The model under review builds one solid part; all positions refer to its coordinate system, in mm. Face numbers are marked on the shaded views. A direction names the side the tool comes from. Round coordinates to 2 decimals unless told otherwise and drop trailing zeros. Write each loop counter-clockwise with the first axis right and the second up, starting at its lowest first coordinate (ties: lowest second). Pieces come first, ordered by that corner, then holes. Notation, with made-up numbers: (76.25, 57) -> (97.25, 57) arc R25 cw to (97.25, 74) -> close; hole circle Ø10 at (-20, 84.25). An arc over 180 degrees is marked (long way). Answer in a Markdown table with one row per item. Add a question column.
```python
from build123d import *

# Parameters (mm, degrees)
SKETCH1_W           = 11.5
SKETCH1_H           = 9
SKETCH1_R           = 1.6
SKETCH1_H_2         = 3
BOSS_EXTRUDE1_DEPTH = 3
SKETCH1_4_W         = 11.5
SKETCH1_4_H         = 3
BOSS_EXTRUDE2_DEPTH = 12
SKETCH1_5_R         = 1.6
CUT_EXTRUDE1_DEPTH  = 2.2
SKETCH1_6_R         = 1.6
CUT_EXTRUDE2_DEPTH  = 21.5
CUT_EXTRUDE3_DEPTH  = 2.2
CUT_EXTRUDE4_DEPTH  = 19.901058171


with BuildPart() as part:
    # Sketch1 → Boss-Extrude1 (new body)
    # profile 1 of 4: a face of its own
    with BuildSketch(Plane(origin=(0, 0, 0), x_dir=(1, 0, 0), z_dir=(0, 1, 0))):
        with Locations((5.75, 7.5)):
            Rectangle(SKETCH1_W, SKETCH1_H)
        Polygon((10.695041723, 7), (8.847520861, 3.8), (5.152479139, 3.8), (3.304958277, 7), (5.152479139, 10.2), (8.847520861, 10.2), align=None, mode=Mode.SUBTRACT)
    # profile 2 of 4: a face of its own
    with BuildSketch(Plane(origin=(0, 0, 0), x_dir=(1, 0, 0), z_dir=(0, 1, 0))):
        Polygon((3.304958277, 7), (5.152479139, 3.8), (8.847520861, 3.8), (10.695041723, 7), (8.847520861, 10.2), (5.152479139, 10.2), align=None)
        with Locations((7, 7)):
            Circle(SKETCH1_R, mode=Mode.SUBTRACT)
    # profile 3 of 4: a face of its own
    with BuildSketch(Plane(origin=(0, 0, 0), x_dir=(1, 0, 0), z_dir=(0, 1, 0))):
        with Locations((7, 7)):
            Circle(SKETCH1_R)
    # profile 4 of 4: a face of its own
    with BuildSketch(Plane(origin=(0, 0, 0), x_dir=(1, 0, 0), z_dir=(0, 1, 0))):
        with Locations((5.75, 1.5)):
            Rectangle(SKETCH1_W, SKETCH1_H_2)
    extrude(amount=BOSS_EXTRUDE1_DEPTH)

    # Sketch1_4 → Boss-Extrude2 (add)
    with BuildSketch(Plane(origin=(0, 0, 0), x_dir=(1, 0, 0), z_dir=(0, 1, 0))):
        with Locations((5.75, 1.5)):
            Rectangle(SKETCH1_4_W, SKETCH1_4_H)
    extrude(amount=-BOSS_EXTRUDE2_DEPTH)

    # Sketch1_5 → Cut-Extrude1 (cut)
    with BuildSketch(Plane(origin=(0, 0, 0), x_dir=(1, 0, 0), z_dir=(0, 1, 0))):
        Polygon((3.304958277, 7), (5.152479139, 3.8), (8.847520861, 3.8), (10.695041723, 7), (8.847520861, 10.2), (5.152479139, 10.2), align=None)
        with Locations(Location((7, 7, 0), (0, 0, 270))):
            Circle(SKETCH1_5_R, mode=Mode.SUBTRACT)
    extrude(amount=CUT_EXTRUDE1_DEPTH, mode=Mode.SUBTRACT)

    # Sketch1_6 → Cut-Extrude2 (cut, through all)
    with BuildSketch(Plane(origin=(0, 0, 0), x_dir=(1, 0, 0), z_dir=(0, 1, 0))):
        with Locations(Location((7, 7, 0), (0, 0, 270))):
            Circle(SKETCH1_6_R)
    extrude(amount=CUT_EXTRUDE2_DEPTH, mode=Mode.SUBTRACT)

    # Sketch3 → Cut-Extrude3 (cut)
    with BuildSketch(Plane(origin=(0, 0, -3), x_dir=(-1, 0, 0), z_dir=(0, 0, -1))):
        with BuildLine():
            Line((-0.304958277, -7), (-2.3, -7))
            ThreePointArc((-2.3, -7), (-4, -8.7), (-5.7, -7))
            Line((-5.7, -7), (-7.695041723, -7))
            Line((-7.695041723, -7), (-5.847520861, -10.2))
            Line((-5.847520861, -10.2), (-2.152479139, -10.2))
            Line((-2.152479139, -10.2), (-0.304958277, -7))
        make_face()
        with BuildLine():
            ThreePointArc((-5.7, -7), (-4, -5.3), (-2.3, -7))
            Line((-2.3, -7), (-0.304958277, -7))
            Line((-0.304958277, -7), (-2.152479139, -3.8))
            Line((-2.152479139, -3.8), (-5.847520861, -3.8))
            Line((-5.847520861, -3.8), (-7.695041723, -7))
            Line((-7.695041723, -7), (-5.7, -7))
        make_face()
    extrude(amount=-CUT_EXTRUDE3_DEPTH, mode=Mode.SUBTRACT)

    # Sketch3_3 → Cut-Extrude4 (cut, through all)
    with BuildSketch(Plane(origin=(0, 0, -3), x_dir=(-1, 0, 0), z_dir=(0, 0, -1))):
        with BuildLine():
            ThreePointArc((-5.7, -7), (-4, -8.7), (-2.3, -7))
            Line((-2.3, -7), (-5.7, -7))
        make_face()
        with BuildLine():
            Line((-5.7, -7), (-2.3, -7))
            ThreePointArc((-2.3, -7), (-4, -5.3), (-5.7, -7))
        make_face()
    extrude(amount=-CUT_EXTRUDE4_DEPTH, mode=Mode.SUBTRACT)


solid = part.part
```
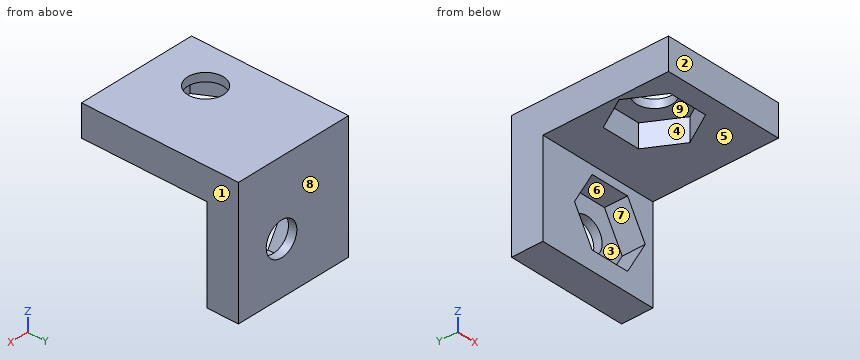
1. Add section A-A on z = -2.5. Write out the cut boundary in (x, y).
2. Add section B-B on y = 1.5. Write out the cut boundary in (x, z).
3. Add section D-D on y = -10. Write out the cut boundary in (x, z), plus the area to 3 significant figures.
4. For L1, parallel to Z at x = 7, y = 2.75; L2, parallel to Y at x = 7.25, z = -9; L3, parallel to Z at x = 5.5, y = 0.25, list the stretches that pass through material, from the lowest coordinate up.
5. Insertion check: pin 1 Ø2 at (x, y) = (6, -2.5) entering from -Z; pin 2 Ø5.5 at (x, y) = (4, -7) entering from -Z; pin 3 Ø3 at (x, z) = (8.5, -7.5) entering from -Y; pin 4 Ø2.5 at (x, z) = (7, -7) entering from -Y. Each pin has a flat end and moves straight along its axis. Give the tip position at first contact, or say it passes through.
6. Mouldability with a two-part tool opening along Z and no side actions: class the marked faces 6, 7, 8 and 9 as pulls with the +Z half, pulls with the -Z half, needs draft (parallel to the pull), parting line crosses it, or undercut.
7. Add section C-C on x = 4. Write out the cut boundary in (y, z), plus the area to 3 significant figures.
8. Tool access review of the marked faces 1, 2, 3, 4 and 5: name each direction out of +Z, -Z, +X, -X, +Y, -Y from which nothing blocks a thin tool from reaching the whole face with its end or side.
Filled in:
| question | item | result |
|---|---|---|
| 1 | outline | (0, -12) -> (11.5, -12) -> (11.5, 3) -> (0, 3) -> close; hole (0.3, -7) -> (2.15, -10.2) -> (5.85, -10.2) -> (7.7, -7) -> (5.85, -3.8) -> (2.15, -3.8) -> close |
| 2 | outline | (0, -12) -> (11.5, -12) -> (11.5, 0) -> (0, 0) -> close; hole (3.3, -7) -> (5.15, -10.2) -> (8.85, -10.2) -> (10.7, -7) -> (8.85, -3.8) -> (5.15, -3.8) -> close |
| 3 | outline | (0, -3) -> (2.04, -3) -> (2.04, -0.8) -> (5.96, -0.8) -> (5.96, -3) -> (11.5, -3) -> (11.5, 0) -> (0, 0) -> close |
| 3 | area | 25.9 mm² |
| 4 | L1 | -12 to -8.6, -5.4 to 0 |
| 4 | L2 | 2.2 to 3 |
| 4 | L3 | -12 to -10.2, -3.8 to 0 |
| 5 | pin 1 | z = -3 |
| 5 | pin 2 | z = -0.8 |
| 5 | pin 3 | y = 2.2 |
| 5 | pin 4 | through |
| 6 | face 6 | undercut |
| 6 | face 7 | undercut |
| 6 | face 8 | needs draft |
| 6 | face 9 | pulls with the -Z half |
| 7 | outline | (-12, -3) -> (-10.2, -3) -> (-10.2, -0.8) -> (-8.7, -0.8) -> (-8.7, 0) -> (-12, 0) -> close; (-5.3, -0.8) -> (-3.8, -0.8) -> (-3.8, -3) -> (0, -3) -> (0, -5.8) -> (2.2, -5.8) -> (2.2, -8.2) -> (0, -8.2) -> (0, -12) -> (3, -12) -> (3, 0) -> (-5.3, 0) -> close |
| 7 | area | 49.9 mm² |
| 8 | face 1 | +Z, -Z, +X, +Y, -Y |
| 8 | face 2 | +Z, -Z, +X, -X, -Y |
| 8 | face 3 | -Y |
| 8 | face 4 | -Z |
| 8 | face 5 | -Z, +X, -X, -Y |
